from build123d import *

# Parameters (mm, degrees)
SKETCH016_W     = 105
SKETCH016_H     = 54
PAD009_DEPTH    = 3
SKETCH028_R     = 3.25
POCKET011_DEPTH = 2
SKETCH029_R     = 3.25
POCKET012_DEPTH = 2
SKETCH030_R     = 3.25
POCKET013_DEPTH = 2


with BuildPart() as part:
    # Sketch016 → Pad009 (new body)
    with BuildSketch(Plane.XY):
        with Locations((0.5, 0)):
            Rectangle(SKETCH016_W, SKETCH016_H)
    extrude(amount=-PAD009_DEPTH)

    # Sketch028 (on Face6 of Pad009) → Pocket011 (cut)
    with BuildSketch(Plane(origin=(0, 0, -3), x_dir=(1, 0, 0), z_dir=(0, 0, -1))):
        with Locations((46.5, 17)):
            Circle(SKETCH028_R)
    extrude(amount=-POCKET011_DEPTH, mode=Mode.SUBTRACT)

    # Sketch029 (on Face5 of Pocket011) → Pocket012 (cut)
    with BuildSketch(Plane(origin=(0, 0, -3), x_dir=(1, 0, 0), z_dir=(0, 0, -1))):
        with Locations((46.5, -17)):
            Circle(SKETCH029_R)
    extrude(amount=-POCKET012_DEPTH, mode=Mode.SUBTRACT)

    # Sketch030 (on Face5 of Pocket012) → Pocket013 (cut)
    with BuildSketch(Plane(origin=(0, 0, -3), x_dir=(1, 0, 0), z_dir=(0, 0, -1))):
        with Locations((-30.2, -1.4)):
            Circle(SKETCH030_R)
    extrude(amount=-POCKET013_DEPTH, mode=Mode.SUBTRACT)


solid = part.part
Source: CAD feature listing. Evaluate the final solid. Frame: model axes, mm. A direction names the side the tool comes from. Round coordinates to 2 decimals unless told otherwise and drop trailing zeros. Write each loop counter-clockwise with the first axis right and the second up, starting at its lowest first coordinate (ties: lowest second). Pieces come first, ordered by that corner, then holes. Notation, with made-up numbers: (15.25, 28.5) - (74.25, 28.5) arc R8 cw to (74.25, 43.5) - close; hole circle Ø10 at (20, 58). An arc over 180 degrees is marked (long way). Use CSV: the item, a comma, the result in double quotes. Start each with the question number.
(1) Set-up query: faces 4 (the face through (0, 27, -1)), 5 (the face through (-30, 1, -1)). Return all of +Z, -Z, +X, -X, +Y, -Y with unobstructed straight access to the full face (end or side cutting, diameter ignored); none if empty.
(2) First-contact query: pin 1 Ø7.5 at (x, y) = (46.5, -17) entering from +Z; pin 2 Ø3 at (x, y) = (46, -18.5) entering from -Z. Flat tips, straight axial feed; report the tip coordinate or a pass-through.
(3) Cut plane B-B, the plane x = 46.5. Return loops of the section in (y, z), and give its area (3 significant figures).
(4) Material intervals for probe 1 along Y at (x, z) = (46.5, -2.45); probe 2 along Y at (x, z) = (-30.2, -2.6); probe 3 along X at (y, z) = (17, -2.2), sorted ascending. Write a range as [from, to].
(5) Cut plane C-C, the plane x = -30.2. Return loops of the section in (y, z), and give its area (3 significant figures).
(6) Mould query, pull axis Y, two halves, no side actions, for faces 1 (the face through (-52, 0, -1)), 2 (the face through (0, -27, -1)), 3 (the face through (-32.595, -0.797, -2.014)). Classes: pulls with the +Y half, pulls with the -Y half, needs draft (parallel to the pull), parting line crosses it, or undercut.
(7) Cut plane A-A, the plane y = 1.4. Return loops of the section in (x, z), and give its area (3 significant figures).
Geometry says:
1,face 4,"+Z, -Z, +X, -X, +Y"
1,face 5,"-Z"
2,pin 1,"z = 0"
2,pin 2,"z = -1"
3,outline,"(-27, -3) - (-20.25, -3) - (-20.25, -1) - (-13.75, -1) - (-13.75, -3) - (13.75, -3) - (13.75, -1) - (20.25, -1) - (20.25, -3) - (27, -3) - (27, 0) - (-27, 0) - close"
3,area,"136 mm²"
4,probe 1,"[-27, -20.25], [-13.75, 13.75], [20.25, 27]"
4,probe 2,"[-27, -1.85], [4.65, 27]"
4,probe 3,"[-52, 43.25], [49.75, 53]"
5,outline,"(-27, -3) - (-1.85, -3) - (-1.85, -1) - (4.65, -1) - (4.65, -3) - (27, -3) - (27, 0) - (-27, 0) - close"
5,area,"149 mm²"
6,face 1,"needs draft"
6,face 2,"pulls with the -Y half"
6,face 3,"undercut"
7,outline,"(-52, -3) - (-33.45, -3) - (-33.45, -1) - (-26.95, -1) - (-26.95, -3) - (53, -3) - (53, 0) - (-52, 0) - close"
7,area,"302 mm²"
